Geometry: see drawing. Coordinates: mm, zero at the bounding-box minimum. A direction names the side the tool comes from. Round coordinates to 2 decimals unless told otherwise and drop trailing zeros. Write each loop counter-clockwise with the first axis right and the second up, starting at its lowest first coordinate (ties: lowest second). Pieces come first, ordered by that corner, then holes.
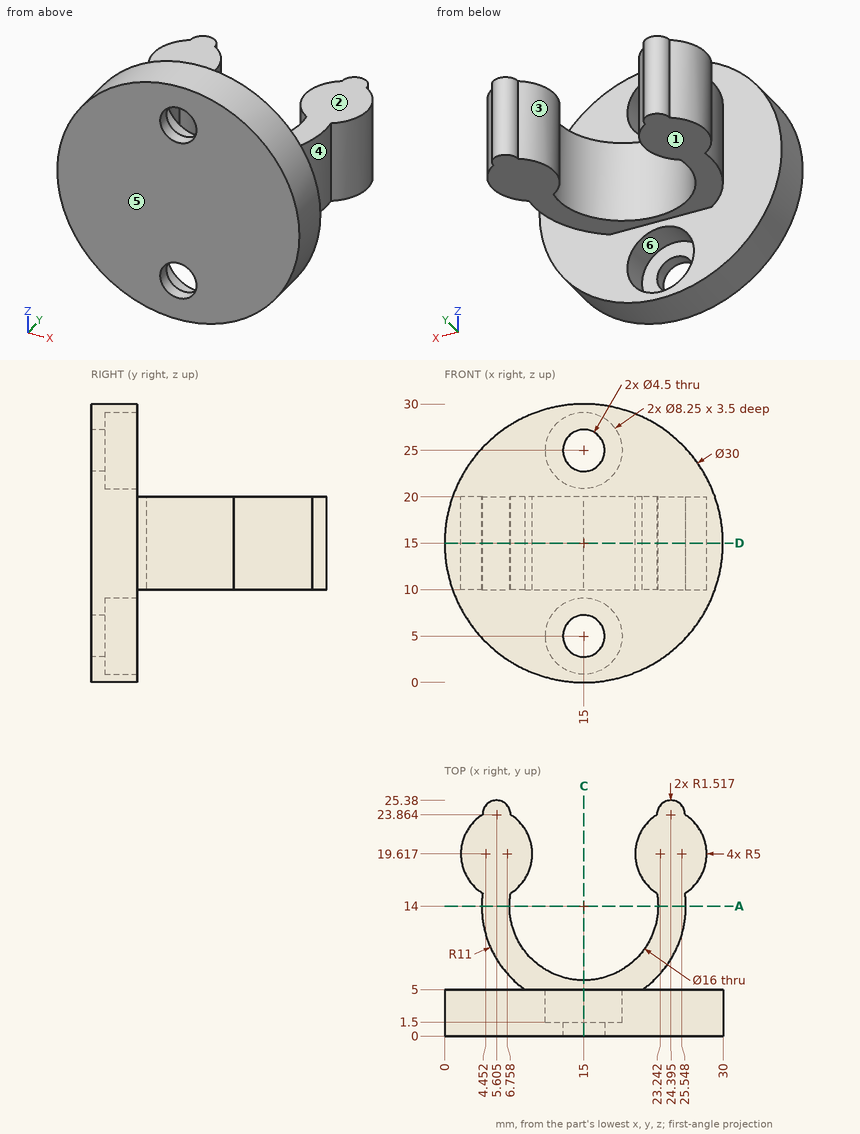
1) Contact query for flat-ended pins moving along their axis: P1, Ø2, axis at y = 7.5, z = 3, coming from the -X side; P2, Ø6, axis at x = 15, z = 25, coming from the -Y side; P3, Ø1, axis at y = 8.5, z = 18.5, coming from the +X side; P4, Ø10.5, axis at x = 15, z = 5, coming from the +Y side. Output: stop coordinate, or through.
Taken from the geometry:
P1: passes through
P2: stops at y = 0
P3: stops at x = 24.8
P4: stops at y = 6.16
2) Section query D-D on z = 15. Return the cut outline in (x, y) (1 decimal), then the cut area to 3 significant figures.
Taken from the geometry:
outline: (0, 0) - (30, 0) - (30, 5) - (21.3, 5) arc R11 ccw to (25.9, 15.4) arc R5 ccw to (25.9, 23.8) arc R1.5 ccw (long way) to (22.9, 23.8) arc R5 ccw to (22.9, 15.4) arc R8 cw (long way) to (7.1, 15.4) arc R5 ccw to (7.1, 23.8) arc R1.5 ccw (long way) to (4.1, 23.8) arc R5 ccw to (4.1, 15.4) arc R11 ccw to (8.7, 5) - (0, 5) - close
area: 345 mm2
3) Section query C-C on x = 15. State how many separate pieces and enclosed holes the cut face has.
Taken from the geometry:
separate pieces: 3
enclosed holes: 0
4) Reachability of the marked faces 1, 2 and 3 from +Z, -Z, +X, -X, +Y, -Y: full face, straight path, thin tool, end or side. Return the list, or none.
Taken from the geometry:
face 1: -Z, +X, -X, +Y
face 2: +Z, +X, -X, +Y
face 3: +Z, -Z
5) Material intervals for line 1 (Z direction, x = 15, y = 0.9); line 2 (X direction, y = 14, z = 15.5); line 3 (Z direction, x = 22.5, y = 20), sorted ascending.
Taken from the geometry:
line 1: z = 0 to 2.75, 7.25 to 22.75, 27.25 to 30
line 2: x = 4 to 7, 23 to 26
line 3: z = 10 to 20
6) Pull-direction query (Y, two-part tool) for the marked faces 4, 5 and 6; classes: released by +Y, released by -Y, zero draft, split by the parting line, or undercut.
Taken from the geometry:
face 4: undercut
face 5: released by -Y
face 6: zero draft
7) Section query A-A on y = 14. Return the cut outline in (x, z).
Taken from the geometry:
outline: (4, 10) - (7, 10) - (7, 20) - (4, 20) - close; (23, 10) - (26, 10) - (26, 20) - (23, 20) - close
